Autodesk Inventor part; units mm, degrees
ref_plane "YZ Plane" through (0, 0, 0) normal (1, 0, 0) x (0, 1, 0)
ref_plane "XZ Plane" through (0, 0, 0) normal (0, 1, 0) x (-1, 0, 0)
ref_plane "XY Plane" through (0, 0, 0) normal (0, 0, 1) x (1, 0, 0)
sketch "Sketch1" plane through (0, 0, 0) normal (0, 0, 1) x (1, 0, 0)
  line L0 (-18.4125, 60.1579) -> (1.5875, 60.1579)
  line L1 (1.5875, 60.1579) -> (1.5875, 34.7579)
  line L2 (1.5875, 34.7579) -> (-18.4125, 34.7579)
  line L3 (-18.4125, 34.7579) -> (-18.4125, 60.1579)
  line L4 (-18.4125, 3.0079) -> (1.5875, 3.0079)
  line L5 (1.5875, 3.0079) -> (1.5875, -22.3921)
  line L6 (1.5875, -22.3921) -> (-18.4125, -22.3921)
  line L7 (-18.4125, -22.3921) -> (-18.4125, 3.0079)
  point P0 (0, 0)
  dimension "d0" = 25.4
  dimension "d1" = 25.4
  dimension "d2" = 20
  dimension "d5" = 31.75
extrude "Extrusion1" add sketch "Sketch1" along normal blind 25.4
sketch "Sketch2" plane through (0, 0, 25.4) normal (0, 0, 1) x (1, 0, 0)
  line L0 (1.5875, 60.1579) -> (-18.4125, 60.1579)
  line L1 (-18.4125, -22.3921) -> (1.5875, -22.3921)
  line L2 (1.5875, 60.1579) -> (-11.9125, 60.1579)
  line L3 (-11.9125, 60.1579) -> (-11.9125, -22.3921)
  line L4 (-11.9125, -22.3921) -> (-4.9125, -22.3921)
  line L5 (-4.9125, -22.3921) -> (-4.9125, 60.1579)
  line L6 (-18.4125, 34.7579) -> (1.5875, 34.7579)
  line L7 (1.5875, 34.7579) -> (1.5875, 60.1579)
  line L8 (1.5875, 60.1579) -> (-18.4125, 60.1579)
  line L9 (-18.4125, 60.1579) -> (-18.4125, 34.7579)
  line L10 (-18.4125, -22.3921) -> (1.5875, -22.3921)
  line L11 (1.5875, -22.3921) -> (1.5875, 3.0079)
  line L12 (1.5875, 3.0079) -> (-18.4125, 3.0079)
  line L13 (-18.4125, 3.0079) -> (-18.4125, -22.3921)
  point P0 (0, 0)
  point P1 (-11.9125, 34.7579)
  point P2 (-11.9125, 3.0079)
  point P3 (-9.9654, 60.1579)
  dimension "d14" = 20
  dimension "d15" = 7
  dimension "d16" = 6.5
extrude "Extrusion2" add sketch "Sketch2" along normal blind 6.35 contours L5 L6 L3 L0 | L5 L12 L3 L6 | L5 L1 L3 L12
sketch "Sketch3" plane through (0, 0, 0) normal (0, 0, -1) x (-1, 0, 0)
  line L0 (4.9125, 3.0079) -> (11.9125, 3.0079)
  line L1 (11.9125, 34.7579) -> (11.9125, 3.0079)
  line L2 (11.9125, 34.7579) -> (4.9125, 34.7579)
  line L3 (4.9125, 3.0079) -> (4.9125, 34.7579)
  line L4 (11.9125, 34.7579) -> (11.9125, 60.1579)
  line L5 (4.9125, 60.1579) -> (4.9125, 34.7579)
  line L6 (11.9125, -22.3921) -> (11.9125, 3.0079)
  line L7 (4.9125, 3.0079) -> (4.9125, -22.3921)
  line L8 (11.9125, 60.1579) -> (4.9125, 60.1579)
  line L9 (-1.5875, 60.1579) -> (18.4125, 60.1579)
  line L10 (11.9125, -22.3921) -> (4.9125, -22.3921)
  line L11 (18.4125, -22.3921) -> (-1.5875, -22.3921)
  point P0 (0, 0)
extrude "Extrusion3" add sketch "Sketch3" along normal blind 6.35
equation "\"d16\" = -0.5 * d15 + 0.5 * d14"
properties part number "spacer_4"
CAD build for the part. Positions are in the model's coordinates, mm. A direction names the side the tool comes from. Coordinates: 2 decimals unless noted, no trailing zeros. Write each loop counter-clockwise with the first axis right and the second up, starting at its lowest first coordinate (ties: lowest second). Pieces come first, ordered by that corner, then holes. Notation, with made-up numbers: (32, 69.25) -> (90, 69.25) arc R28 cw to (90, 90.25) -> close; hole circle Ø6 at (23.25, 7). An arc over 180 degrees is marked (long way). Use CSV: the item, a comma, the result in double quotes. Start each with the question number.
Item 1: Band-saw the part on D-D, the plane y = 48. Write the cut outline in (x, z), plus the area to 3 significant figures.
Item 2: Band-saw the part on B-B, the plane z = 6.5. Write the cut outline in (x, y), plus the area to 3 significant figures.
Item 3: Wall check: probe 1 along Y at (x, z) = (-17, 6.5); probe 2 along Z at (x, y) = (-8.5, 16); probe 3 along X at (y, z) = (-18, 30). Give the ranges that are in metal, low to high.
Item 4: Two-plate mould, pull along Z, no slides. Class faces 1 (the flat face through (-15, -10, 0)), 2 (the flat face through (-9, 3.008, 13)), 3 (the flat face through (-11.912, 19, -3)): +Z half, -Z half, draft (parallel to the pull), parting line (faces both ways), or undercut.
Item 5: Band-saw the part on C-C, the plane x = -10.75. Write the cut outline in (y, z), plus the area to 3 significant figures.
Item 6: Tool access for faces 4 (the flat face through (-8, 34.758, 13)), 5 (the flat face through (-15, 48, 0)), 6 (the flat face through (-2, 48, 25.4)), 7 (the flat face through (-2, -10, 0)), 8 (the flat face through (-11.912, 19, 29)): list every direction of +Z, -Z, +X, -X, +Y, -Y with a clear straight run to the whole face (end or side of a thin tool).
Item 7: Drop flat-ended pins along their axis: P1, Ø1.9, axis at y = 15.5, z = -2.5, coming from the +X side; P2, Ø1.9, axis at y = 11, z = -2, coming from the -X side; P3, Ø3.5, axis at x = -16.5, y = -16, coming from the +Z side. Give the stop position or say it passes through.
Item 8: Band-saw the part on A-A, the plane x = -16.5. Write the cut outline in (y, z).
Response values:
1,outline,"(-18.41, 0) -> (-11.91, 0) -> (-11.91, -6.35) -> (-4.91, -6.35) -> (-4.91, 0) -> (1.59, 0) -> (1.59, 25.4) -> (-4.91, 25.4) -> (-4.91, 31.75) -> (-11.91, 31.75) -> (-11.91, 25.4) -> (-18.41, 25.4) -> close"
1,area,"597 mm2"
2,outline,"(-18.41, -22.39) -> (1.59, -22.39) -> (1.59, 3.01) -> (-18.41, 3.01) -> close; (-18.41, 34.76) -> (1.59, 34.76) -> (1.59, 60.16) -> (-18.41, 60.16) -> close"
2,area,"1,020 mm2"
3,probe 1,"y = -22.39 to 3.01, 34.76 to 60.16"
3,probe 2,"z = -6.35 to 0, 25.4 to 31.75"
3,probe 3,"x = -11.91 to -4.91"
4,face 1,"-Z half"
4,face 2,"undercut"
4,face 3,"draft"
5,outline,"(-22.39, -6.35) -> (60.16, -6.35) -> (60.16, 31.75) -> (-22.39, 31.75) -> close; hole (3.01, 0) -> (34.76, 0) -> (34.76, 25.4) -> (3.01, 25.4) -> close"
5,area,"2,340 mm2"
6,face 4,"+X, -X"
6,face 5,"-Z, -X, +Y, -Y"
6,face 6,"+Z, +X, +Y, -Y"
6,face 7,"-Z, +X, +Y, -Y"
6,face 8,"+Z, -X, +Y, -Y"
7,P1,"stops at x = -4.91"
7,P2,"stops at x = -11.91"
7,P3,"stops at z = 25.4"
8,outline,"(-22.39, 0) -> (3.01, 0) -> (3.01, 25.4) -> (-22.39, 25.4) -> close; (34.76, 0) -> (60.16, 0) -> (60.16, 25.4) -> (34.76, 25.4) -> close"
